```python
from build123d import *

# Parameters (mm, degrees)
F0_W     = 50.8
F0_H     = 76.2
F1_DEPTH = 127
F5_R     = 5.08


with BuildPart() as f1:
    # F0 (on Front) → F1 (new body)
    with BuildSketch(Plane.XZ):
        with Locations((0, -38.1)):
            Rectangle(F0_W, F0_H)
    extrude(amount=-F1_DEPTH)

    # F4: sweep along a path in F2
    with BuildLine(Plane.YZ) as f4_path:
        CenterArc((63.5, 245.9344424842), 254, 0, 360)
    # F3 (on Front) → F4 (sweep, cut)
    with BuildSketch(Plane.XZ):
        with BuildLine():
            Line((1.3198227154, -19.7110452561), (12.7, 0))
            Line((12.7, 0), (43.4110164642, 0))
            Line((43.4110164642, 0), (43.4110164642, 26.4454465359))
            Line((43.4110164642, 26.4454465359), (-29.6869948506, 26.4454465359))
            Line((-29.6869948506, 26.4454465359), (-29.6869948506, 0))
            Line((-29.6869948506, 0), (-12.7, 0))
            Line((-12.7, 0), (-1.3198227154, -19.7110452561))
            ThreePointArc((-1.3198227154, -19.7110452561), (0, -20.4730452561), (1.3198227154, -19.7110452561))
        make_face()
    sweep(path=f4_path.line, mode=Mode.SUBTRACT)

    # F5
    f5_edges = [f1.edges().sort_by_distance(p)[0] for p in [
        (-12.7, 63.5, -8.065558),
        (12.7, 63.5, -8.065558),
    ]]
    fillet(f5_edges, radius=F5_R)


solid = f1.part
```
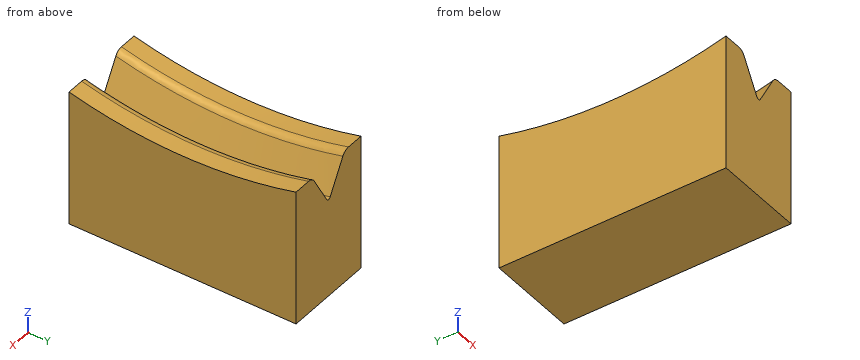
Read the model definition and answer for the solid it produces. Units are mm, in the model's axes. Round coordinates to 2 decimals unless told otherwise and drop trailing zeros. Write each loop counter-clockwise with the first axis right and the second up, starting at its lowest first coordinate (ties: lowest second). Pieces come first, ordered by that corner, then holes. Notation, with made-up numbers: (31.5, 41.25) -> (64.5, 41.25) arc R33 cw to (64.5, 70.25) -> close; hole circle Ø1 at (-29, 77.5). An arc over 180 degrees is marked (long way). Answer in a Markdown table with one row per item. Add a question column.
1) Find section A-A, the plane x = -20.5. Determine the outline of the cut face in (y, z), and give its area (3 significant figures).
2) Given P1, Ø8, axis at x = 9, y = 63.5, coming from the +Z side; P2, Ø1.5, axis at x = -1.5, y = 108, coming from the +Z side, each flat-ended and moving along its own axis, determine where each tip first touches the part or whether it passes through.
3) Consider line 1 (X direction, y = 116.5, z = -21); line 2 (X direction, y = 39, z = -26); line 3 (Z direction, x = 13.5, y = 80.5). Determine where each line is inside the solid, lowest interval first.
Findings below:
| question | item | result |
|---|---|---|
| 1 | outline | (0, -76.2) -> (127, -76.2) -> (127, 0) arc R254 cw to (0, 0) -> close |
| 1 | area | 8,990 mm² |
| 2 | P1 | z = -8.77 |
| 2 | P2 | z = -21.95 |
| 3 | line 1 | -25.4 to -1.9, 1.9 to 25.4 |
| 3 | line 2 | -25.4 to -1.38, 1.38 to 25.4 |
| 3 | line 3 | -76.2 to -7.95 |
